```python
from build123d import *

# Parameters (mm, degrees)
SKETCH1_W           = 40
SKETCH1_H           = 40
BOSS_EXTRUDE1_DEPTH = 9
SKETCH2_W           = 40
SKETCH2_H           = 9
BOSS_EXTRUDE2_DEPTH = 31
SKETCH3_W           = 8.5
SKETCH3_H           = 19.5
CUT_EXTRUDE1_DEPTH  = 42.964270517
SKETCH4_W           = 8.5
SKETCH4_H           = 19.5
CUT_EXTRUDE2_DEPTH  = 55.415071442
BOSS_EXTRUDE3_DEPTH = 5
BOSS_EXTRUDE4_DEPTH = 5
CHAMFER1_SIZE       = 1


with BuildPart() as part:
    # Sketch1 → Boss-Extrude1 (new body)
    with BuildSketch(Plane(origin=(0, 0, 0), x_dir=(1, 0, 0), z_dir=(0, 1, 0))):
        Rectangle(SKETCH1_W, SKETCH1_H)
    extrude(amount=BOSS_EXTRUDE1_DEPTH)

    # Sketch2 → Boss-Extrude2 (add)
    with BuildSketch(Plane(origin=(0, 9, 0), x_dir=(1, 0, 0), z_dir=(0, 1, 0))):
        with Locations((0, 15.5)):
            Rectangle(SKETCH2_W, SKETCH2_H)
    extrude(amount=BOSS_EXTRUDE2_DEPTH)

    # Sketch3 → Cut-Extrude1 (cut, through all)
    with BuildSketch(Plane(origin=(0, 9, 0), x_dir=(1, 0, 0), z_dir=(0, 1, 0))):
        with Locations((0, -5.25)):
            Rectangle(SKETCH3_W, SKETCH3_H)
    extrude(amount=-CUT_EXTRUDE1_DEPTH, mode=Mode.SUBTRACT)

    # Sketch4 → Cut-Extrude2 (cut, through all)
    with BuildSketch(Plane.XY.offset(-11)):
        with Locations((0, 25.25)):
            Rectangle(SKETCH4_W, SKETCH4_H)
    extrude(amount=-CUT_EXTRUDE2_DEPTH, mode=Mode.SUBTRACT)

    # Sketch5 → Boss-Extrude3 (add)
    with BuildSketch(Plane.ZY.offset(20)):
        Polygon((-11, 40), (20, 9), (-11, 9), align=None)
    extrude(amount=-BOSS_EXTRUDE3_DEPTH)

    # Sketch6 → Boss-Extrude4 (add)
    with BuildSketch(Plane(origin=(20, 0, 0), x_dir=(0, 0, -1), z_dir=(1, 0, 0))):
        Polygon((-20, 9), (11, 40), (11, 9), align=None)
    extrude(amount=-BOSS_EXTRUDE4_DEPTH)

    # Chamfer1
    chamfer1_edges = [part.edges().sort_by_distance(p)[0] for p in [
        (0, 40, -20),
        (0, 0, 20),
    ]]
    chamfer(chamfer1_edges, length=CHAMFER1_SIZE)


solid = part.part
```
Design review of the part built by this model. Coordinates are the model's own, in mm. A direction names the side the tool comes from. Coordinates: 2 decimals unless noted, no trailing zeros. Loops run counter-clockwise (first coordinate to the right, second up) from the corner with the lowest first, then second, coordinate; pieces in that order, holes last. Notation, with made-up numbers: (-13, 6.5) -> (41, 6.5) arc R14 ccw to (41, 29.5) -> close; hole circle Ø7 at (49, 36.25). An arc over 180 degrees is marked (long way). Answer as a JSON object with one key per item and string values.
Q1. Take a section at C-C on y = 5. Give the boundary of the cut face in (x, z).
Answer block:
{"outline": "(-20, -20) -> (20, -20) -> (20, 20) -> (-20, 20) -> close; hole (-4.25, -4.5) -> (4.25, -4.5) -> (4.25, 15) -> (-4.25, 15) -> close"}
Q2. To check wall thickness, follow L1, parallel to X at y = 11, z = -2; L2, parallel to X at y = 33, z = -18; L3, parallel to Z at x = -10, y = 13.5. State the ranges of each line that lie inside material, in increasing order.
Answer block:
{"L1": "x = -20 to -15, 15 to 20", "L2": "x = -20 to -4.25, 4.25 to 20", "L3": "z = -20 to -11"}
Q3. Tool access review of faces 4 (the flat face through (-7, 24, -11)), 5 (the flat face through (0, 35, -15)), 6 (the flat face through (0, 5, -4.5)): name each direction out of +Z, -Z, +X, -X, +Y, -Y from which nothing blocks a thin tool from reaching the whole face with its end or side.
Answer block:
{"face 4": "+Z, +Y", "face 5": "+Z, -Z", "face 6": "+Y, -Y"}
Q4. Take a section at A-A on y = 17.5. Give the boundary of the cut face in (x, z), plus the area to 4 significant figures.
Answer block:
{"outline": "(-20, -20) -> (-4.25, -20) -> (-4.25, -11) -> (-15, -11) -> (-15, 11.5) -> (-20, 11.5) -> close; (4.25, -20) -> (20, -20) -> (20, 11.5) -> (15, 11.5) -> (15, -11) -> (4.25, -11) -> close", "area": "508.5 mm^2"}
Q5. Take a section at B-B on z = -0.5. Give the boundary of the cut face in (x, y).
Answer block:
{"outline": "(-20, 0) -> (-4.25, 0) -> (-4.25, 9) -> (-15, 9) -> (-15, 29.5) -> (-20, 29.5) -> close; (4.25, 0) -> (20, 0) -> (20, 29.5) -> (15, 29.5) -> (15, 9) -> (4.25, 9) -> close"}
Q6. Clearance check with a flat-ended pin moving along its axis: pin 1 Ø10 at (x, y) = (5.5, 31) entering from +Z. State where the tip first meets the part, or that it passes through.
Answer block:
{"pin 1": "stops at z = -11"}
Q7. The part is to be moulded in two halves that separate along Z. For faces 1 (the flat face through (-18, 25, 4)), 2 (the flat face through (0, 5, 15)), 3 (the flat face through (-15, 18, -2)), say which applies: +Z half, -Z half, draft (parallel to the pull), parting line (faces both ways), or undercut.
Answer block:
{"face 1": "+Z half", "face 2": "undercut", "face 3": "draft"}
Q8. Take a section at D-D on z = -12.5. Give the boundary of the cut face in (x, y).
Answer block:
{"outline": "(-20, 0) -> (20, 0) -> (20, 40) -> (-20, 40) -> close; hole (-4.25, 15.5) -> (4.25, 15.5) -> (4.25, 35) -> (-4.25, 35) -> close"}
